CAD build for the part. Positions are in the model's coordinates, mm. A direction names the side the tool comes from. Coordinates: 2 decimals unless noted, no trailing zeros. Loops run counter-clockwise (first coordinate to the right, second up) from the corner with the lowest first, then second, coordinate; pieces in that order, holes last. Notation, with made-up numbers: (-24.5, -2.5) - (22.5, -2.5) arc R14 cw to (22.5, 2.5) - close; hole circle Ø11 at (62, -39). An arc over 180 degrees is marked (long way). Put each result on its own line as item: value.
```python
from build123d import *

# Parameters (mm, degrees)
SKETCH1_W           = 104
SKETCH1_H           = 145
BOSS_EXTRUDE1_DEPTH = 10
SKETCH2_W           = 104
SKETCH2_H           = 2
CUT_EXTRUDE1_DEPTH  = 3
FILLET2_R           = 5


with BuildPart() as part:
    # Sketch1 → Boss-Extrude1 (new body)
    with BuildSketch(Plane(origin=(0, 0, 0), x_dir=(1, 0, 0), z_dir=(0, 1, 0))):
        Rectangle(SKETCH1_W, SKETCH1_H)
    extrude(amount=BOSS_EXTRUDE1_DEPTH)

    # Sketch2 → Cut-Extrude1 (cut)
    with BuildSketch(Plane(origin=(0, 10, 0), x_dir=(1, 0, 0), z_dir=(0, 1, 0))):
        with Locations((0, 66.5)):
            Rectangle(SKETCH2_W, SKETCH2_H)
        with Locations((0, -63.5)):
            Rectangle(SKETCH2_W, SKETCH2_H)
    extrude(amount=-CUT_EXTRUDE1_DEPTH, mode=Mode.SUBTRACT)

    # Fillet2
    fillet2_edges = [part.edges().sort_by_distance(p)[0] for p in [
        (0, 10, 72.5),
    ]]
    fillet(fillet2_edges, radius=FILLET2_R)


solid = part.part
```
Q1. Tool access for faces 4 (the flat face through (-1, 9, -67.5)), 5 (the flat face through (-1, 10, -2)): list every direction of +Z, -Z, +X, -X, +Y, -Y with a clear straight run to the whole face (end or side of a thin tool).
Determined:
face 4: +X, -X, +Y
face 5: +Z, -Z, +X, -X, +Y
Q2. Wall check: L1, parallel to Z at x = -9, y = 9; L2, parallel to Z at x = 11.5, y = 8.5. Give the ranges that are in metal, low to high. Write a range as from..to.
Determined:
L1: -72.5..-67.5, -65.5..62.5, 64.5..70.5
L2: -72.5..-67.5, -65.5..62.5, 64.5..71.07
Q3. Mould opens along Z. For faces 1 (the flat face through (-1, 9, 62.5)), 2 (the cylindrical face through (0.73, 8.57, 71)), 3 (the flat face through (-1, 10, -70)) say: +Z half, -Z half, draft (parallel to the pull), parting line (faces both ways), or undercut.
Determined:
face 1: undercut
face 2: +Z half
face 3: draft
Q4. Pin check, flat tips, straight feed: pin 1 Ø3.5 at (x, y) = (-25, 8) entering from +Z; pin 2 Ø2.5 at (x, y) = (-12, 8.5) entering from +Z. Stop position of each tip, or through.
Determined:
pin 1: z = 72.34
pin 2: z = 71.97
Q5. Slice it at A-A, the plane y = 8.5. Give the cut face in (x, z), then the cut area to 3 significant figures.
Determined:
outline: (-52, -72.5) - (52, -72.5) - (52, -67.5) - (-52, -67.5) - close; (-52, -65.5) - (52, -65.5) - (52, 62.5) - (-52, 62.5) - close; (-52, 64.5) - (52, 64.5) - (52, 71.07) - (-52, 71.07) - close
area: 14,500 mm2
